CAD build for the part. Positions are in the model's coordinates, mm. Face numbers are marked on the shaded views. A direction names the side the tool comes from. Round coordinates to 2 decimals unless told otherwise and drop trailing zeros. Order: outer loops, then holes, each group sorted by start corner. A loop starts at its lowest first (then second) coordinate and runs counter-clockwise, first axis right, second up. Notation, with made-up numbers: M 78.25,17.25 L 96.25,17.25 A31 ccw 96.25,55.25 Z; hole C 50,-37.5 d10. An arc over 180 degrees is marked long. Answer as a JSON object with one key per item and string values.
```python
from build123d import *

# Parameters (mm, degrees)
SKETCH_1_W          = 50
SKETCH_1_H          = 55
EXTRUDE_1_DEPTH     = 30
EXTRUDE_2_DEPTH     = 10
SKETCH_3_R          = 2
CUT_EXTRUDE_1_DEPTH = 10


with BuildPart() as part:
    # 草图1 → 凸台-拉伸1 (new body, symmetric)
    with BuildSketch(Plane.XY):
        Rectangle(SKETCH_1_W, SKETCH_1_H)
    extrude(amount=EXTRUDE_1_DEPTH, both=True)

    # 草图2 → 凸台-拉伸2 (add)
    with BuildSketch(Plane(origin=(0, 0, -30), x_dir=(-1, 0, 0), z_dir=(0, 0, -1))):
        with BuildLine():
            Line((11.180339887, 10), (-11.180339887, 10))
            ThreePointArc((-11.180339887, 10), (0, -15), (11.180339887, 10))
        make_face()
    extrude(amount=EXTRUDE_2_DEPTH)

    # 草图3 → 切除-拉伸1 (cut)
    with BuildSketch(Plane(origin=(0, 27.5, 0), x_dir=(1, 0, 0), z_dir=(0, 1, 0))):
        Circle(SKETCH_3_R)
    extrude(amount=-CUT_EXTRUDE_1_DEPTH, mode=Mode.SUBTRACT)


solid = part.part
```
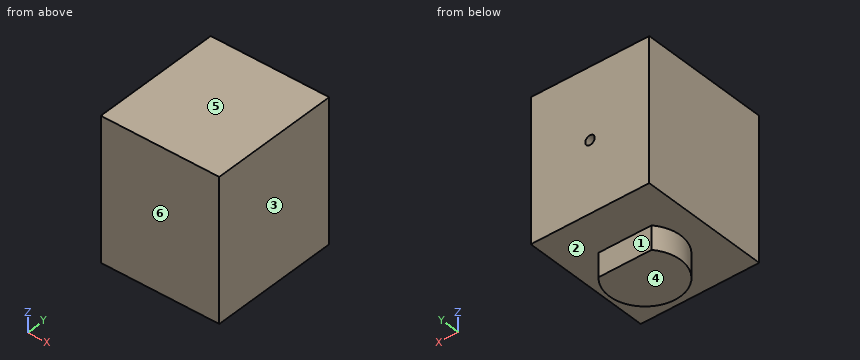
Item 1: Saw through at C-C on x = 9.5. List the corners of the cut face in (y, z), and give its area (3 significant figures).
Worked answers:
{"outline": "M -27.5,-30 L -11.61,-30 L -11.61,-40 L 10,-40 L 10,-30 L 27.5,-30 L 27.5,30 L -27.5,30 Z", "area": "3,520 mm2"}
Item 2: Wall check: line 1 along Z through (x, y) = (0, 24); line 2 along X through (y, z) = (20.5, 0); line 3 along Z through (x, y) = (-9.5, 22.5). Give the ranges that are in metal, low to high. Write a range as [from, to].
Worked answers:
{"line 1": "z = [-30, -2], [2, 30]", "line 2": "x = [-25, -2], [2, 25]", "line 3": "z = [-30, 30]"}
Item 3: Saw through at D-D on x = 18.5. List the corners of the cut face in (y, z).
Worked answers:
{"outline": "M -27.5,-30 L 27.5,-30 L 27.5,30 L -27.5,30 Z"}
Item 4: 3-axis set-ups, long thin cutter, end or side, ignore diameter. For the marked faces 1, 2 and 3: which of +Z, -Z, +X, -X, +Y, -Y reach the whole face in a straight line?
Worked answers:
{"face 1": "-Z, +X, -X, +Y", "face 2": "-Z", "face 3": "+Z, -Z, +X, +Y, -Y"}
Item 5: Two-plate mould, pull along Z, no slides. Class the marked faces 4, 5 and 6: released by +Z, released by -Z, zero draft, split by the parting line, or undercut.
Worked answers:
{"face 4": "released by -Z", "face 5": "released by +Z", "face 6": "zero draft"}
Item 6: Drop flat-ended pins along their axis: pin 1 Ø1.5 at (x, y) = (-12.5, 19.5) entering from -Z; pin 2 Ø8 at (x, z) = (2.5, -37.5) entering from +Y; pin 3 Ø4.5 at (x, z) = (0.5, 0) entering from +Y. Give the stop position or say it passes through.
Worked answers:
{"pin 1": "stops at z = -30", "pin 2": "stops at y = 10", "pin 3": "stops at y = 27.5"}
Item 7: Saw through at B-B on x = 0. List the corners of the cut face in (y, z), and give its area (3 significant figures).
Worked answers:
{"outline": "M -27.5,-30 L -15,-30 L -15,-40 L 10,-40 L 10,-30 L 27.5,-30 L 27.5,-2 L 17.5,-2 L 17.5,2 L 27.5,2 L 27.5,30 L -27.5,30 Z", "area": "3,510 mm2"}
Item 8: Saw through at A-A on y = 0. List the corners of the cut face in (x, z).
Worked answers:
{"outline": "M -25,-30 L -15,-30 L -15,-40 L 15,-40 L 15,-30 L 25,-30 L 25,30 L -25,30 Z"}
